The model under review builds one solid part; all positions refer to its coordinate system, in mm. A direction names the side the tool comes from. Round coordinates to 2 decimals unless told otherwise and drop trailing zeros. Loops run counter-clockwise (first coordinate to the right, second up) from the corner with the lowest first, then second, coordinate; pieces in that order, holes last. Notation, with made-up numbers: M 58,52.5 L 83,52.5 A26 ccw 83,85.5 Z; hole C 64.25,0 d4. An arc over 180 degrees is marked long. Use a Markdown table: item, result. Add a question column.
```python
from build123d import *

# Parameters (mm, degrees)
SKETCH1_W           = 190.5
SKETCH1_H           = 50.8
BOSS_EXTRUDE1_DEPTH = 25.4
SKETCH2_W           = 63.5
SKETCH2_H           = 228.6
BOSS_EXTRUDE2_DEPTH = 50.8
SKETCH3_W           = 190.5
SKETCH3_H           = 50.8
BOSS_EXTRUDE3_DEPTH = 6.35
SKETCH4_R           = 22.225
CUT_EXTRUDE1_DEPTH  = 307.712230764
SKETCH5_W           = 50.8
SKETCH5_H           = 254
BOSS_EXTRUDE4_DEPTH = 6.35
LPATTERN2_START     = 203.2
LPATTERN2_OUTLINE_R = 22.225
LPATTERN2_DEPTH     = 50.8
SKETCH6_W           = 190.5
SKETCH6_H           = 50.8
BOSS_EXTRUDE5_DEPTH = 25.4


# Read off the part's stored shape, not the designer's step: LPattern2
with BuildPart() as part:
    # Sketch1 → Boss-Extrude1 (new body)
    with BuildSketch(Plane.XY):
        with Locations((95.25, 25.4)):
            Rectangle(SKETCH1_W, SKETCH1_H)
    extrude(amount=BOSS_EXTRUDE1_DEPTH)

    # Sketch2 → Boss-Extrude2 (add)
    with BuildSketch(Plane.XZ):
        with Locations((120.65, -114.3)):
            Rectangle(SKETCH2_W, SKETCH2_H)
    extrude(amount=-BOSS_EXTRUDE2_DEPTH)

    # Sketch3 → Boss-Extrude3 (add)
    with BuildSketch(Plane(origin=(0, 0, -228.6), x_dir=(-1, 0, 0), z_dir=(0, 0, -1))):
        with Locations((-95.25, 25.4)):
            Rectangle(SKETCH3_W, SKETCH3_H)
    extrude(amount=BOSS_EXTRUDE3_DEPTH)

    # Sketch4 → Cut-Extrude1 (cut, through all)
    with BuildSketch(Plane.XZ):
        with Locations(Location((120.65, -143.027799697, 0), (0, 0, 270))):
            Circle(SKETCH4_R)
    extrude(amount=-CUT_EXTRUDE1_DEPTH, mode=Mode.SUBTRACT)

    # Sketch5 → Boss-Extrude4 (add)
    with BuildSketch(Plane.ZY.offset(-88.9)):
        with Locations((-133.35, 127)):
            Rectangle(SKETCH5_W, SKETCH5_H)
    extrude(amount=BOSS_EXTRUDE4_DEPTH)

    # LPattern2 outline → LPattern2 (add)
    with BuildSketch(Plane(origin=(0, 0, 0), x_dir=(1, 0, 0), z_dir=(0, 1, 0)).offset(LPATTERN2_START)):
        Polygon((88.9, 228.6), (88.9, 0), (152.4, 0), (152.4, 228.6), (190.5, 228.6), (190.5, 234.95), (0, 234.95), (0, 228.6), align=None)
        with Locations((120.65, 143.027799697)):
            Circle(LPATTERN2_OUTLINE_R, mode=Mode.SUBTRACT)
    extrude(amount=LPATTERN2_DEPTH)

    # Sketch6 → Boss-Extrude5 (add)
    with BuildSketch(Plane.XY):
        with Locations((95.25, 228.6)):
            Rectangle(SKETCH6_W, SKETCH6_H)
    extrude(amount=BOSS_EXTRUDE5_DEPTH)


solid = part.part
```
(1) Consider section B-B, the plane z = -190. Give the boundary of the cut face in (x, y), then the cut area to 3 significant figures.
(2) Consider section A-A, the plane x = 147.5. Give the boundary of the cut face in (y, z), then the cut area to 3 significant figures.
(3) Consider section C-C, the plane x = 23.5. Give the boundary of the cut face in (y, z), then the cut area to 3 significant figures.
(4) Consider section D-D, the plane z = -129.5. Give the boundary of the cut face in (x, y), then the cut area to 3 significant figures.
(5) Insertion check: pin 1 Ø6 at (x, z) = (83, -201) entering from -Y; pin 2 Ø5 at (y, z) = (120, -125) entering from +X; pin 3 Ø4 at (y, z) = (216.5, -77.5) entering from -X; pin 4 Ø15 at (y, z) = (219.5, -76) entering from +X. Each pin has a flat end and moves straight along its axis. Give the tip position at first contact, or say it passes through.
(6) Draft analysis for pull direction Y (two halves, no side actions). For faces 4 (the face through (115, 254, -78)), 5 (the face through (86, 125, -158.75)), 6 (the face through (118, 50.8, -74)), 7 (the face through (118, 0, -78)), state which applies: released by +Y, released by -Y, zero draft, split by the parting line, or undercut.
(7) To check wall thickness, follow probe 1 along Y at (x, z) = (147.5, -50); probe 2 along Z at (x, y) = (120, 234); probe 3 along Z at (x, y) = (23, 21.5). State the ranges of each line that lie inside material, in increasing order.
(8) For faces 1 (the face through (44, 229, 0)), 2 (the face through (130.905, 228.244, -123.31)), 3 (the face through (172, 26, -228.6)), list the 3-axis set-ups (+Z, -Z, +X, -X, +Y, -Y) from which the entire face can be reached by the end or side of a thin tool; tool diameter is ignored.
Found:
| question | item | result |
|---|---|---|
| 1 | outline | M 88.9,0 L 152.4,0 L 152.4,50.8 L 88.9,50.8 Z; M 88.9,203.2 L 152.4,203.2 L 152.4,254 L 88.9,254 Z |
| 1 | area | 6,450 mm^2 |
| 2 | outline | M 0,-234.95 L 50.8,-234.95 L 50.8,25.4 L 0,25.4 Z; M 203.2,-234.95 L 254,-234.95 L 254,25.4 L 203.2,25.4 Z |
| 2 | area | 26,500 mm^2 |
| 3 | outline | M 0,-234.95 L 50.8,-234.95 L 50.8,-228.6 L 0,-228.6 Z; M 0,0 L 50.8,0 L 50.8,25.4 L 0,25.4 Z; M 203.2,-234.95 L 254,-234.95 L 254,-228.6 L 203.2,-228.6 Z; M 203.2,0 L 254,0 L 254,25.4 L 203.2,25.4 Z |
| 3 | area | 3,230 mm^2 |
| 4 | outline | M 82.55,0 L 103.02,0 L 103.02,50.8 L 88.9,50.8 L 88.9,203.2 L 103.02,203.2 L 103.02,254 L 82.55,254 Z; M 138.28,0 L 152.4,0 L 152.4,50.8 L 138.28,50.8 Z; M 138.28,203.2 L 152.4,203.2 L 152.4,254 L 138.28,254 Z |
| 4 | area | 4,480 mm^2 |
| 5 | pin 1 | passes through |
| 5 | pin 2 | stops at x = 88.9 |
| 5 | pin 3 | stops at x = 88.9 |
| 5 | pin 4 | stops at x = 152.4 |
| 6 | face 4 | released by +Y |
| 6 | face 5 | zero draft |
| 6 | face 6 | undercut |
| 6 | face 7 | released by -Y |
| 7 | probe 1 | y = 0 to 50.8, 203.2 to 254 |
| 7 | probe 2 | z = -234.95 to -165.24, -120.81 to 25.4 |
| 7 | probe 3 | z = -234.95 to -228.6, 0 to 25.4 |
| 8 | face 1 | -X, +Y, -Y |
| 8 | face 2 | +Y, -Y |
| 8 | face 3 | +X, +Y, -Y |
